from build123d import *
from build123d.topology import SkipClean

# Parameters (mm, degrees)
SKETCH_1_R             = 0.75
EXTRUDE_1_DEPTH        = 2
SKETCH_2_R             = 0.8
SKETCH_4_R             = 1
EXTRUDE_2_DEPTH        = 1.55
SKETCH_5_W             = 9.9
SKETCH_5_H             = 5
EXTRUDE_3_DEPTH        = 9
SKETCH_8_R             = 0.4
EXTRUDE_5_DEPTH        = 2
EXTRUDE_5_2_DEPTH      = 2
SKETCH_9_W             = 2.7
SKETCH_9_H             = 1.7
EXTRUDE_6_DEPTH        = 4
CUT_EXTRUDE_3_DEPTH    = 7
SKETCH_7_R             = 1.25
EXTRUDE_7_DEPTH        = 6
PATTERN_LINEAR_1_COUNT = 2
PATTERN_LINEAR_1_PITCH = 5
EXTRUDE_8_DEPTH        = 7
FILLET_1_R             = 0.5
FILLET_2_R             = 0.5
FILLET_4_R             = 0.5
FILLET_5_R             = 0.5


with BuildPart() as part:
    # Sketch 1 → Extrude 1 (new body)
    with BuildSketch(Plane.XY):
        Circle(SKETCH_1_R)
    extrude_1 = extrude(amount=-EXTRUDE_1_DEPTH)

    # Sweep 1: sweep along a path in Sketch 3
    with BuildLine(Plane(origin=(0, 0, 0), x_dir=(0, 0, -1), z_dir=(1, 0, 0))) as sweep_1_path:
        ThreePointArc((0, 0), (-1.838477631, 0.761522369), (-2.6, 2.6))
    # Sketch 2 → Sweep 1 (sweep)
    with BuildSketch(Plane.XY):
        Circle(SKETCH_2_R)
    sweep_1 = sweep(path=sweep_1_path.line)

    # Sketch 4 → Extrude 2 (add)
    with BuildSketch(Plane(origin=(0, 2.6, 0), x_dir=(1, 0, 0), z_dir=(0, 1, 0))):
        with Locations(Location((0, -2.6, 0), (0, 0, 90))):
            Circle(SKETCH_4_R)
    extrude_2 = extrude(amount=EXTRUDE_2_DEPTH)

    # Sketch 5 → Extrude 3 (add)
    with BuildSketch(Plane(origin=(0, 4.15, 0), x_dir=(1, 0, 0), z_dir=(0, 1, 0))):
        with Locations((-2.5, -2.6)):
            Rectangle(SKETCH_5_W, SKETCH_5_H)
    extrude(amount=EXTRUDE_3_DEPTH)



with BuildPart() as body_2:
    # Sketch 8 → Extrude 5 (new body)
    with BuildSketch(Plane.XY):
        with Locations((-8, 10)):
            Circle(SKETCH_8_R)
    extrude(amount=-EXTRUDE_5_DEPTH)


with BuildPart() as body_3:
    # Sketch 8 → Extrude 5 2 (new body)
    with BuildSketch(Plane.XY):
        with Locations((3, 10)):
            Circle(SKETCH_8_R)
    extrude(amount=-EXTRUDE_5_2_DEPTH)


with BuildPart() as part_1:
    add(part.part)

    add(body_2.part)  # Extrude 6 merges body 2

    add(body_3.part)  # Extrude 6 merges body 3
    # Sketch 9 → Extrude 6 (add)
    with BuildSketch(Plane.XY):
        with Locations((-7.8, 10)):
            Rectangle(SKETCH_9_W, SKETCH_9_H)
        with Locations((2.8, 10)):
            Rectangle(SKETCH_9_W, SKETCH_9_H)
    extrude(amount=EXTRUDE_6_DEPTH)

    # Sketch 6 → Cut-Extrude 3 (cut)
    with BuildSketch(Plane(origin=(0, 13.15, 0), x_dir=(1, 0, 0), z_dir=(0, 1, 0))):
        with BuildLine():
            Line((0, -0.6), (-7, -0.6))
            Line((-7, -0.6), (-7, -4.6))
            Line((-7, -4.6), (0, -4.6))
            ThreePointArc((0, -4.6), (2, -2.6), (0, -0.6))
        make_face()
    extrude(amount=-CUT_EXTRUDE_3_DEPTH, mode=Mode.SUBTRACT)

    # Sketch 7 → Extrude 7 (add)
    with BuildSketch(Plane(origin=(0, 6.15, 0), x_dir=(1, 0, 0), z_dir=(0, 1, 0))):
        with Locations(Location((0, -2.6, 0), (0, 0, 90))):
            Circle(SKETCH_7_R)
    extrude_7 = extrude(amount=EXTRUDE_7_DEPTH)

    # Pattern Linear 1: Extrude 1, Sweep 1, Extrude 2, Extrude 7 ×2
    with Locations(*[(-i * PATTERN_LINEAR_1_PITCH, 0, 0) for i in range(1, PATTERN_LINEAR_1_COUNT)]):
        add(extrude_1)
        add(sweep_1)
        add(extrude_2)
        add(extrude_7)

    # Sketch 10 → Extrude 8 (add)
    with BuildSketch(Plane(origin=(0, 13.15, 0), x_dir=(1, 0, 0), z_dir=(0, 1, 0))):
        with BuildLine():
            Line((-5, -0.6), (0, -0.6))
            ThreePointArc((0, -0.6), (-1.028991511, -0.885014149), (-1.764705882, -1.658823529))
            ThreePointArc((-1.764705882, -1.658823529), (-2.5, -2.1), (-3.235294118, -1.658823529))
            ThreePointArc((-3.235294118, -1.658823529), (-3.971008489, -0.885014149), (-5, -0.6))
        make_face()
    extrude_8 = extrude(amount=-EXTRUDE_8_DEPTH)

    # Mirror 2: Extrude 8 across plane
    with SkipClean():  # the faces are left unmerged after this step: merging them gives an invalid solid
        add(extrude_8.mirror(Plane(origin=(0, 0, 2.6), x_dir=(1, 0, 0), z_dir=(0, 0, -1))))

    # Fillet 1
    fillet_1_edges = [part_1.edges().sort_by_distance(p)[0] for p in [
        (-9.15, 9.15, 2),
        (-9.15, 10.85, 2),
        (4.15, 10.85, 2),
        (4.15, 9.15, 2),
    ]]
    fillet(fillet_1_edges, radius=FILLET_1_R)

    # Fillet 2
    fillet_2_edges = [part_1.edges().sort_by_distance(p)[0] for p in [
        (-7.45, 8.65, 5.1),
        (2.45, 8.65, 5.1),
    ]]
    fillet(fillet_2_edges, radius=FILLET_2_R)

    # Fillet 4
    fillet_4_edges = [part_1.edges().sort_by_distance(p)[0] for p in [
        (-7, 9.65, 4.6),
        (-7, 9.65, 0.6),
    ]]
    fillet(fillet_4_edges, radius=FILLET_4_R)

    # Fillet 5
    fillet_5_edges = [part_1.edges().sort_by_distance(p)[0] for p in [
        (0, 12.15, 3.85),
        (-5, 12.15, 3.85),
    ]]
    fillet(fillet_5_edges, radius=FILLET_5_R)


solid = part_1.part
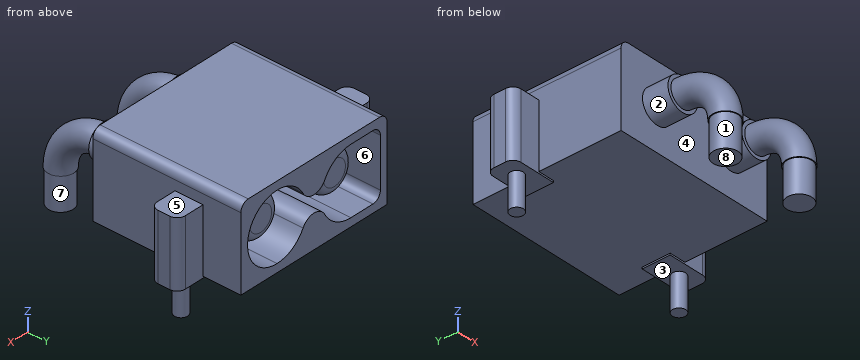
Geometry: final body of the model. Coordinates: model frame, mm. Face numbers are marked on the shaded views. A direction names the side the tool comes from. Coordinates: 2 decimals unless noted, no trailing zeros. Order: outer loops, then holes, each group sorted by start corner. A loop starts at its lowest first (then second) coordinate and runs counter-clockwise, first axis right, second up. Notation, with made-up numbers: M 11,-26.5 L 42,-26.5 A28 ccw 42,6.5 Z; hole C -2,-2 d6. An arc over 180 degrees is marked long. One line per question, with ' | ' between items. Start each with the question number.
Item 1: Cut plane D-D, the plane y = 10. Count the separate pieces of the cut face and the enclosed holes in it, then the cut area to 3 significant figures.
Item 2: Ray query, probe 1 along X at (y, z) = (10, 2.25); probe 2 along X at (y, z) = (6.5, 3); probe 3 along X at (y, z) = (6.75, 4.25). Return the intervals inside material, ascending. Write a range as [from, to].
Item 3: Set-up query: the marked faces 4, 5, 6, 7 and 8. Return all of +Z, -Z, +X, -X, +Y, -Y with unobstructed straight access to the full face (end or side cutting, diameter ignored); none if empty.
Item 4: Cut plane C-C, the plane x = 3. Return the cut outline in (y, z).
Item 5: Draft query along Y for the marked faces 1, 2 and 3. Return one class per face: released by +Y, released by -Y, zero draft, split by the parting line, or undercut.
Item 6: Pin query (flat end, axial travel): pin 1 Ø0.6 at (x, z) = (0.5, 3) entering from -Y; pin 2 Ø0.7 at (x, z) = (-7.5, 2) entering from -Y; pin 3 Ø0.5 at (x, y) = (2, 10) entering from -Z. Return the tip coordinate at first contact, or that it passes through.
Item 7: Cut plane B-B, the plane z = -0.5. Return the cut outline in (x, y), then the cut area to 3 significant figures.
Item 8: Cut plane A-A, the plane y = 7. Return the cut outline in (x, z), then the cut area to 3 significant figures.
A:
1) separate pieces: 3 | enclosed holes: 1 | area: 48.2 mm2
2) probe 1: x = [-9.15, -7], [-6.2, -3.8], [-1.2, 1.2], [1.97, 4.15] | probe 2: x = [-7.45, -7], [-6.18, -3.82], [-1.18, 1.18], [1.96, 2.45] | probe 3: x = [-7.45, -6.98], [-3.87, -1.13], [1.13, 2.45]
3) face 4: none | face 5: +Z, +X, +Y, -Y | face 6: +Y | face 7: -Z | face 8: -Z, +X, -X, +Y, -Y
4) outline: M 9.15,0 L 9.6,0 L 9.6,-2 L 10.4,-2 L 10.4,0 L 10.85,0 L 10.85,4 L 9.15,4 Z
5) face 1: split by the parting line | face 2: undercut | face 3: zero draft
6) pin 1: stops at y = 0.73 | pin 2: stops at y = 4.15 | pin 3: stops at z = 0
7) outline: C -8,10 d0.8; C -5,0 d1.5; C 0,0 d1.5; C 3,10 d0.8 | area: 4.54 mm2
8) outline: M -7.45,0.1 L 2.45,0.1 L 2.45,4.6 A0.5 ccw 1.95,5.1 L -6.95,5.1 A0.5 ccw -7.45,4.6 Z; C -5,2.6 d2.5; C 0,2.6 d2.5; hole M -7,1.1 A0.5 ccw -6.5,0.6 L -5,0.6 A2 ccw -3.24,1.66 A0.83 cw -1.76,1.66 A2 ccw long -1.76,3.54 A0.83 cw -3.24,3.54 A2 ccw -5,4.6 L -6.5,4.6 A0.5 ccw -7,4.1 Z | area: 31.2 mm2
